Here's how the part is built. I have some questions about the finished solid (model axes, mm). A direction names the side the tool comes from. Round coordinates to 2 decimals unless told otherwise and drop trailing zeros. Loops run counter-clockwise (first coordinate to the right, second up) from the corner with the lowest first, then second, coordinate; pieces in that order, holes last. Notation, with made-up numbers: (-29, 0.25) - (23, 0.25) arc R15 ccw to (23, 14.25) - close; hole circle Ø1 at (-0.5, 43.5). An arc over 180 degrees is marked (long way). Answer as a JSON object with one key per item and string values. Group by question number.
1) If we mould it in two halves opening along X, with no side actions, what happens to faces 1 (the face through (28, 112, 3)), 2 (the face through (-1.891, 95, 3)), 3 (the face through (7, 147, 0))? For each: pulls with the +X half, pulls with the -X half, needs draft (parallel to the pull), parting line crosses it, or undercut.
2) I want a section at A-A, the plane y = 91. Please give me the cut outline in (x, z), then the cut area to 3 significant figures.
3) Which directions (+Z, -Z, +X, -X, +Y, -Y) give clear straight access to the entire face, cutting with the end or side of a thin tool? Please do faces 4 (the face through (13, 71.985, 3)), 5 (the face through (22, -25, 3)).
4) Will these pins go through, and if not, where does the flat tip stop? P1, Ø1.8, axis at x = 11, z = 3, coming from the -Y side; P2, Ø2.5, axis at x = -3.39, y = 128, coming from the -Z side.
5) If I drill on line 1 along X through (y, z) = (128, 4.4); line 2 along X through (y, z) = (63, 2.25); line 3 along Y through (x, z) = (-17, 5) (3 decimals), over which ranges is the centre line in solid material (lowest first)? Write a range as [from, to].
6) I want a section at B-B, the plane z = 3.25. Give the number of separate pieces and of enclosed holes in the cut face, then the cut area to 3 significant figures.
from build123d import *

# Parameters (mm, degrees)
SKETCH_1_W            = 67
SKETCH_1_H            = 30
EXTRUDE_1_DEPTH       = 6
SKETCH_3_R            = 11.5
CUT_EXTRUDE_1_DEPTH   = 7
CUT_EXTRUDE_2_DEPTH   = 35
EXTRUDE_2_DEPTH       = 6
FILLET_1_R            = 2.5
FILLET_3_R            = 0.5
FILLET_4_R            = 7
SKETCH_6_R            = 2
CUT_EXTRUDE_3_DEPTH   = 7
EXTRUDE_3_DEPTH       = 6
CUT_EXTRUDE_4_DEPTH   = 7
EXTRUDE_4_DEPTH       = 6
SKETCH_10_R           = 2.1
CUT_EXTRUDE_5_DEPTH   = 7
FILLET_5_R            = 5
SKETCH_11_R           = 1.6
CUT_EXTRUDE_6_DEPTH   = 7
CUT_EXTRUDE_7_DEPTH   = 10
FILLET_6_R            = 2
SKETCH_13_OUTSIDE_W   = 121.737
SKETCH_13_OUTSIDE_H   = 129.266
SKETCH_13_OUTSIDE_W_2 = 53.782400736
SKETCH_13_OUTSIDE_H_2 = 120
CUT_EXTRUDE_8_DEPTH   = 10
EXTRUDE_5_DEPTH       = 6
SKETCH_15_W           = 53.782400736
SKETCH_15_H           = 178
EXTRUDE_6_DEPTH       = 6
SKETCH_16_R           = 1.525
CUT_EXTRUDE_9_DEPTH   = 10
SKETCH_17_W           = 3.06
SKETCH_17_H           = 50.06
CUT_EXTRUDE_10_DEPTH  = 6
SKETCH_18_R           = 1.505
CUT_EXTRUDE_11_DEPTH  = 6
SKETCH_19_R           = 1.525
CUT_EXTRUDE_12_DEPTH  = 6
SKETCH_20_W           = 17.891200368
SKETCH_20_H           = 45.985
CUT_EXTRUDE_13_DEPTH  = 10
FILLET_7_R            = 2


with BuildPart() as part:
    # 草图1 → 凸台-拉伸1 (new body)
    with BuildSketch(Plane.XY):
        Rectangle(SKETCH_1_W, SKETCH_1_H)
    extrude(amount=EXTRUDE_1_DEPTH)

    # 草图3 → 切除-拉伸1 (cut, through all)
    with BuildSketch(Plane.XY.offset(6)):
        with Locations((0.155997342, -18.5)):
            Circle(SKETCH_3_R)
    extrude(amount=-CUT_EXTRUDE_1_DEPTH, mode=Mode.SUBTRACT)

    # 草图4 → 切除-拉伸2 (cut)
    with BuildSketch(Plane.XY.offset(6)):
        with BuildLine():
            Line((14.951296016, -3.246749948), (0.155997342, -34.975370344))
            Line((0.155997342, -34.975370344), (0.155997342, -27))
            Line((0.155997342, -27), (-20.283732192, -12.687947301))
            ThreePointArc((-20.283732192, -12.687947301), (-5.343907366, 2.025923809), (14.951296016, -3.246749948))
        make_face()
    extrude(amount=-CUT_EXTRUDE_2_DEPTH, mode=Mode.SUBTRACT)

    # 草图5 → 凸台-拉伸2 (add)
    with BuildSketch(Plane.XY.offset(6)):
        Polygon((-16.981778738, -15), (-2.700298671, -25), (-33.5, -25), (-33.5, -15), align=None)
        Polygon((33.5, -15), (33.5, -25), (4.807588927, -25), (10.334473164, -13.147558505), align=None)
    extrude(amount=-EXTRUDE_2_DEPTH)

    # 圆角1
    fillet_1_edges = [part.edges().sort_by_distance(p)[0] for p in [
        (-2.700298671, -25, 3),
    ]]
    fillet(fillet_1_edges, radius=FILLET_1_R)

    # 圆角3
    fillet_3_edges = [part.edges().sort_by_distance(p)[0] for p in [
        (-20.283732192, -12.687947301, 3),
        (14.951296016, -3.246749948, 3),
    ]]
    fillet(fillet_3_edges, radius=FILLET_3_R)

    # 圆角4
    fillet_4_edges = [part.edges().sort_by_distance(p)[0] for p in [
        (4.807588927, -25, 3),
    ]]
    fillet(fillet_4_edges, radius=FILLET_4_R)

    # 草图6 → 切除-拉伸3 (cut, through all)
    with BuildSketch(Plane.XY.offset(6)):
        with Locations((17.505658254, -13.841257188)):
            Circle(SKETCH_6_R)
        with Locations((-17.782400736, -20.381512339)):
            Circle(SKETCH_6_R)
    extrude(amount=-CUT_EXTRUDE_3_DEPTH, mode=Mode.SUBTRACT)

    # 草图7 → 凸台-拉伸3 (add)
    with BuildSketch(Plane.XY.offset(6)):
        Polygon((60.5, 75), (14.5, 75), (-16.303792618, 15), (33.5, 15), align=None)
    extrude(amount=-EXTRUDE_3_DEPTH)

    # 草图8 → 切除-拉伸4 (cut, through all)
    with BuildSketch(Plane.XY.offset(6)):
        Polygon((-16.303792618, 15), (-33.5, -18.49498082), (-33.5, 15), align=None)
    extrude(amount=-CUT_EXTRUDE_4_DEPTH, mode=Mode.SUBTRACT)

    # 草图9 → 凸台-拉伸4 (add)
    with BuildSketch(Plane.XY.offset(6)):
        Polygon((60.5, 75), (33.5, -25), (33.5, 15), align=None)
    extrude(amount=-EXTRUDE_4_DEPTH)

    # 草图10 → 切除-拉伸5 (cut, through all)
    with BuildSketch(Plane.XY.offset(6)):
        with Locations((-12, 10)):
            Circle(SKETCH_10_R)
        with Locations((23, 10)):
            Circle(SKETCH_10_R)
    extrude(amount=-CUT_EXTRUDE_5_DEPTH, mode=Mode.SUBTRACT)

    # 圆角5
    fillet_5_edges = [part.edges().sort_by_distance(p)[0] for p in [
        (60.5, 75, 3),
        (14.5, 75, 3),
    ]]
    fillet(fillet_5_edges, radius=FILLET_5_R)

    # 草图11 → 切除-拉伸6 (cut, through all)
    with BuildSketch(Plane.XY.offset(6)):
        with Locations((42.500000039, 67)):
            Circle(SKETCH_11_R)
        with Locations((22.500000039, 67)):
            Circle(SKETCH_11_R)
    extrude(amount=-CUT_EXTRUDE_6_DEPTH, mode=Mode.SUBTRACT)

    # 草图12 → 切除-拉伸7 (cut)
    with BuildSketch(Plane.XY.offset(6)):
        Polygon((33.412019277, 64), (31.452414539, 20), (29.670955687, -20), (52.350955687, 64), align=None)
        Polygon((28.047412755, 55.924590701), (-1.630833947, 20), (26.447458252, 20), align=None)
        Polygon((14.473082867, 64), (-8.116365053, 20), (28.233189094, 64), align=None)
    extrude(amount=-CUT_EXTRUDE_7_DEPTH, mode=Mode.SUBTRACT)

    # 圆角6
    fillet_6_edges = [part.edges().sort_by_distance(p)[0] for p in [
        (29.670955687, -20, 3),
        (33.412019277, 64, 3),
        (52.350955687, 64, 3),
        (14.473082867, 64, 3),
        (28.233189094, 64, 3),
        (-8.116365053, 20, 3),
        (28.047412755, 55.924590701, 3),
        (26.447458252, 20, 3),
        (-1.630833947, 20, 3),
    ]]
    fillet(fillet_6_edges, radius=FILLET_6_R)

    # 草图13 outside → 切除-拉伸8 (cut)
    with BuildSketch(Plane.XY.offset(6)):
        with Locations((12.7355, 25)):
            Rectangle(SKETCH_13_OUTSIDE_W, SKETCH_13_OUTSIDE_H)
        with Locations((1.108799632, 35)):
            Rectangle(SKETCH_13_OUTSIDE_W_2, SKETCH_13_OUTSIDE_H_2, mode=Mode.SUBTRACT)
    extrude(amount=-CUT_EXTRUDE_8_DEPTH, mode=Mode.SUBTRACT)

    # 草图14 → 凸台-拉伸5 (add)
    with BuildSketch(Plane.XY.offset(6)):
        Polygon((-25.782400736, -3.462547587), (-25.782400736, 75), (28, 75), (28, 15), (-16.303792618, 15), align=None)
    extrude(amount=-EXTRUDE_5_DEPTH)

    # 草图15 → 凸台-拉伸6 (add)
    with BuildSketch(Plane.XY.offset(6)):
        with Locations((1.108799632, 164)):
            Rectangle(SKETCH_15_W, SKETCH_15_H)
    extrude(amount=-EXTRUDE_6_DEPTH)

    # 草图16 → 切除-拉伸9 (cut)
    with BuildSketch(Plane.XY.offset(6)):
        with Locations((-7, 250)):
            Circle(SKETCH_16_R)
        with Locations((13, 250)):
            Circle(SKETCH_16_R)
    extrude(amount=-CUT_EXTRUDE_9_DEPTH, mode=Mode.SUBTRACT)

    # 草图17 → 切除-拉伸10 (cut)
    with BuildSketch(Plane.XY.offset(6)):
        with Locations((1.108799632, 148)):
            Rectangle(SKETCH_17_W, SKETCH_17_H)
    extrude(amount=-CUT_EXTRUDE_10_DEPTH, mode=Mode.SUBTRACT)

    # 草图18 → 切除-拉伸11 (cut)
    with BuildSketch(Plane.XY.offset(6)):
        with Locations((2.638799632, 124.475)):
            Circle(SKETCH_18_R)
        with Locations((-0.421200368, 124.475)):
            Circle(SKETCH_18_R)
        with Locations((-0.421200368, 171.525)):
            Circle(SKETCH_18_R)
        with Locations((2.638799632, 171.525)):
            Circle(SKETCH_18_R)
    extrude(amount=-CUT_EXTRUDE_11_DEPTH, mode=Mode.SUBTRACT)

    # 草图19 → 切除-拉伸12 (cut)
    with BuildSketch(Plane.XY.offset(6)):
        with Locations((-3.391200368, 148)):
            Circle(SKETCH_19_R)
        with Locations((-3.391200368, 128)):
            Circle(SKETCH_19_R)
    extrude(amount=-CUT_EXTRUDE_12_DEPTH, mode=Mode.SUBTRACT)

    # 草图20 → 切除-拉伸13 (cut)
    with BuildSketch(Plane.XY.offset(6)):
        with Locations((13.054399816, 94.9775)):
            Rectangle(SKETCH_20_W, SKETCH_20_H)
        with Locations((13.054399816, 42.9925)):
            Rectangle(SKETCH_20_W, SKETCH_20_H)
        with Locations((-10.836800552, 42.9925)):
            Rectangle(SKETCH_20_W, SKETCH_20_H)
        with Locations((-10.836800552, 94.9775)):
            Rectangle(SKETCH_20_W, SKETCH_20_H)
        Polygon((1.108799632, 207.860027008), (-18.392920488, 178.03), (20.610519752, 178.03), align=None)
        Polygon((23, 241.345027008), (3.49827988, 211.515), (23, 181.684972992), align=None)
        Polygon((-20.782400736, 241.345027008), (-20.782400736, 181.684972992), (-1.280680616, 211.515), align=None)
        Polygon((-18.392920488, 245), (1.108799632, 215.169972992), (20.610519752, 245), align=None)
    extrude(amount=-CUT_EXTRUDE_13_DEPTH, mode=Mode.SUBTRACT)

    # 圆角7
    fillet_7_edges = [part.edges().sort_by_distance(p)[0] for p in [
        (4.108799632, 65.985, 3),
        (22, 65.985, 3),
        (22, 20, 3),
        (4.108799632, 20, 3),
        (-1.891200368, 65.985, 3),
        (-1.891200368, 20, 3),
        (-19.782400736, 20, 3),
        (-19.782400736, 65.985, 3),
        (-19.782400736, 71.985, 3),
        (-19.782400736, 117.97, 3),
        (-1.891200368, 117.97, 3),
        (-1.891200368, 71.985, 3),
        (1.108799632, 207.860027008, 3),
        (20.610519752, 178.03, 3),
        (-18.392920488, 178.03, 3),
        (-18.392920488, 245, 3),
        (20.610519752, 245, 3),
        (1.108799632, 215.169972992, 3),
        (-20.782400736, 181.684972992, 3),
        (-20.782400736, 241.345027008, 3),
        (-1.280680616, 211.515, 3),
        (3.49827988, 211.515, 3),
        (23, 241.345027008, 3),
        (23, 181.684972992, 3),
        (4.108799632, 117.97, 3),
        (22, 117.97, 3),
        (22, 71.985, 3),
        (4.108799632, 71.985, 3),
    ]]
    fillet(fillet_7_edges, radius=FILLET_7_R)


solid = part.part
Outcome:
{
 "1": {"face 1": "pulls with the +X half", "face 2": "undercut", "face 3": "needs draft"},
 "2": {"outline": "(-25.78, 0) - (-19.78, 0) - (-19.78, 6) - (-25.78, 6) - close; (-1.89, 0) - (4.11, 0) - (4.11, 6) - (-1.89, 6) - close; (22, 0) - (28, 0) - (28, 6) - (22, 6) - close", "area": "108 mm^2"},
 "3": {"face 4": "+Z, -Z", "face 5": "+Z, -Z, +X, -X, -Y"},
 "4": {"P1": "y = -23.82", "P2": "through"},
 "5": {"line 1": "[-25.78, -4.92], [-1.87, -0.42], [2.64, 28]", "line 2": "[-25.78, -19.78], [-1.89, 4.11], [22, 28]", "line 3": "[-25, -22.222], [-18.541, -14.987], [-5.961, 20], [65.985, 71.985], [117.97, 187.471], [235.559, 253]"},
 "6": {"separate pieces": "1", "enclosed holes": "17", "area": "8,460 mm^2"}
}
